from build123d import *

# Parameters (mm, degrees)
SCHIZZO1_W                   = 15
SCHIZZO1_H                   = 76.1
ESTRUSIONE_ESTRUSIONE1_DEPTH = 11
SCHIZZO2_W                   = 15
SCHIZZO2_H                   = 8.2
ESTRUSIONE_ESTRUSIONE2_DEPTH = 62.5
SCHIZZO3_R                   = 7.5
ESTRUSIONE_ESTRUSIONE3_DEPTH = 8.2
SCHIZZO4_R                   = 4
ESTRUSIONE_ESTRUSIONE4_DEPTH = 7
SMUSSO1_SIZE                 = 0.5
SCHIZZO5_W                   = 15
SCHIZZO5_H                   = 8.2
ESTRUSIONE_ESTRUSIONE5_DEPTH = 70
F_3_0_3_DIAMETER_HOLE1_D     = 3
F_3_0_3_DIAMETER_HOLE1_DEPTH = 10
F_3_0_3_DIAMETER_HOLE1_TIP   = 0.901290929
RACCORDO1_R                  = 7.5
RACCORDO2_R                  = 7
F_4_0_4_DIAMETER_HOLE1_D     = 4
SCHIZZO12_R                  = 4.5
ESTRUSIONE_ESTRUSIONE6_DEPTH = 1
F_3_0_3_DIAMETER_HOLE2_D     = 3
F_3_0_3_DIAMETER_HOLE2_DEPTH = 8.2


with BuildPart() as part:
    # Schizzo1 → Estrusione-Estrusione1 (new body)
    with BuildSketch(Plane.XY):
        with Locations((7.5, 38.05)):
            Rectangle(SCHIZZO1_W, SCHIZZO1_H)
    extrude(amount=ESTRUSIONE_ESTRUSIONE1_DEPTH)

    # Schizzo2 → Estrusione-Estrusione2 (add)
    with BuildSketch(Plane.XY.offset(11)):
        with Locations((7.5, 4.1)):
            Rectangle(SCHIZZO2_W, SCHIZZO2_H)
    extrude(amount=ESTRUSIONE_ESTRUSIONE2_DEPTH)

    # Schizzo3 → Estrusione-Estrusione3 (add)
    with BuildSketch(Plane(origin=(0, 8.2, 0), x_dir=(1, 0, 0), z_dir=(0, 1, 0))):
        with Locations((7.5, -73.5)):
            Circle(SCHIZZO3_R)
    extrude(amount=-ESTRUSIONE_ESTRUSIONE3_DEPTH)

    # Schizzo4 → Estrusione-Estrusione4 (add)
    with BuildSketch(Plane(origin=(0, 8.2, 0), x_dir=(1, 0, 0), z_dir=(0, 1, 0))):
        with Locations(Location((7.5, -73.5, 0), (0, 0, 90))):
            Circle(SCHIZZO4_R)
    extrude(amount=ESTRUSIONE_ESTRUSIONE4_DEPTH)

    # Smusso1
    smusso1_edges = [part.edges().sort_by_distance(p)[0] for p in [
        (7.5, 15.2, 77.5),
    ]]
    chamfer(smusso1_edges, length=SMUSSO1_SIZE)

    # Schizzo5 → Estrusione-Estrusione5 (add)
    with BuildSketch(Plane.XY.offset(11)):
        with Locations((7.5, 72)):
            Rectangle(SCHIZZO5_W, SCHIZZO5_H)
    extrude(amount=ESTRUSIONE_ESTRUSIONE5_DEPTH)

    # Ø3.0 (3) Diameter Hole1
    with Locations(Plane(origin=(0, 76.1, 0), x_dir=(1, 0, 0), z_dir=(0, 1, 0))):
        with Locations((7.5, -49.5), (7.5, -53.5)):
            Hole(F_3_0_3_DIAMETER_HOLE1_D / 2, depth=F_3_0_3_DIAMETER_HOLE1_DEPTH)
            with Locations((0, 0, -(F_3_0_3_DIAMETER_HOLE1_DEPTH + F_3_0_3_DIAMETER_HOLE1_TIP / 2))):  # 118° drill point
                Cone(0, F_3_0_3_DIAMETER_HOLE1_D / 2, F_3_0_3_DIAMETER_HOLE1_TIP, mode=Mode.SUBTRACT)

    # Raccordo1
    raccordo1_edges = [part.edges().sort_by_distance(p)[0] for p in [
        (15, 72, 81),
        (0, 72, 81),
    ]]
    fillet(raccordo1_edges, radius=RACCORDO1_R - 0.0001)  # a hair under: the kernel refuses the full size

    # Raccordo2
    raccordo2_edges = [part.edges().sort_by_distance(p)[0] for p in [
        (7.5, 76.1, 0),
        (7.5, 0, 0),
    ]]
    fillet(raccordo2_edges, radius=RACCORDO2_R)

    # Ø4.0 (4) Diameter Hole1 (through all)
    with Locations(Plane(origin=(15, 0, 0), x_dir=(0, 0, -1), z_dir=(1, 0, 0))):
        with Locations((-5.5, 19.8), (-5.5, 47.8)):
            Hole(F_4_0_4_DIAMETER_HOLE1_D / 2)

    # Schizzo12 → Estrusione-Estrusione6 (add)
    with BuildSketch(Plane(origin=(0, 8.2, 0), x_dir=(1, 0, 0), z_dir=(0, 1, 0))):
        with Locations(Location((7.5, -73.5, 0), (0, 0, 90))):
            Circle(SCHIZZO12_R)
    extrude(amount=ESTRUSIONE_ESTRUSIONE6_DEPTH)

    # Ø3.0 (3) Diameter Hole2
    with Locations(Plane(origin=(0, 76.1, 0), x_dir=(1, 0, 0), z_dir=(0, 1, 0))):
        with Locations((7.5, -73.5)):
            Hole(F_3_0_3_DIAMETER_HOLE2_D / 2, depth=F_3_0_3_DIAMETER_HOLE2_DEPTH)


solid = part.part
For this review, take the finished solid that the model builds, in its own axes (mm). A direction names the side the tool comes from. Coordinates: 2 decimals unless noted, no trailing zeros. Loops run counter-clockwise (first coordinate to the right, second up) from the corner with the lowest first, then second, coordinate; pieces in that order, holes last. Notation, with made-up numbers: (72.25, -36) - (105.25, -36) arc R16 cw to (105.25, -8) - close; hole circle Ø2 at (-33.5, 2). An arc over 180 degrees is marked (long way). Use a Markdown table: item, result. Add a question column.
Item 1: Insertion check: pin 1 Ø8 at (x, y) = (3, 51) entering from +Z. The pin has a flat end and moves straight along its axis. Give the tip position at first contact, or say it passes through.
Item 2: We need section B-B (z = 26.5). Give the boundary of the cut face in (x, y), and give its area (3 significant figures).
Item 3: We need section D-D (x = 1.75). Give the boundary of the cut face in (y, z), and give its area (3 significant figures).
Item 4: Tool access review of faces 4 (the face through (7.825, 71.943, 50.964)), 5 (the face through (7, 0, 43)), 6 (the face through (7, 15.2, 74)), 7 (the face through (10, 9.2, 77)), 8 (the face through (7.395, 49.783, 5.24)): name each direction out of +Z, -Z, +X, -X, +Y, -Y from which nothing blocks a thin tool from reaching the whole face with its end or side.
Item 5: For line 1 (Y direction, x = 9, z = 20.5); line 2 (X direction, y = 70, z = 49.5); line 3 (Z direction, x = 7.5, y = 70.25), list the stretches that pass through material, from the lowest coordinate up.
Item 6: We need section C-C (z = 49.5). Give the boundary of the cut face in (x, y).
Item 7: Mouldability with a two-part tool opening along Z and no side actions: class faces 1 (the face through (7, 67.9, 46)), 2 (the face through (6.694, 71.943, 72.235)), 3 (the face through (7.34, 4.16, 81)) as pulls with the +Z half, pulls with the -Z half, needs draft (parallel to the pull), parting line crosses it, or undercut.
Item 8: We need section A-A (y = 47.8). Give the boundary of the cut face in (x, z).
Results list:
| question | item | result |
|---|---|---|
| 1 | pin 1 | stops at z = 11 |
| 2 | outline | (0, 0) - (15, 0) - (15, 8.2) - (0, 8.2) - close; (0, 67.9) - (15, 67.9) - (15, 76.1) - (0, 76.1) - close |
| 2 | area | 246 mm^2 |
| 3 | outline | (0, 7) arc R7 ccw to (7, 0) - (69.1, 0) arc R7 ccw to (76.1, 7) - (76.1, 78.32) - (67.9, 78.32) - (67.9, 11) - (8.2, 11) - (8.2, 78.32) - (0, 78.32) - close; hole circle Ø4 at (19.8, 5.5); hole circle Ø4 at (47.8, 5.5) |
| 3 | area | 1,890 mm^2 |
| 4 | face 4 | +Y |
| 4 | face 5 | +Z, -Z, +X, -X, -Y |
| 4 | face 6 | +Z, +X, -X |
| 4 | face 7 | none |
| 4 | face 8 | +X, -X |
| 5 | line 1 | y = 0 to 8.2, 67.9 to 76.1 |
| 5 | line 2 | x = 0 to 6, 9 to 15 |
| 5 | line 3 | z = 0.1 to 48, 51 to 52, 55 to 72, 75 to 81 |
| 6 | outline | (0, 0) - (15, 0) - (15, 8.2) - (0, 8.2) - close; (0, 67.9) - (6, 67.9) - (6, 76.1) - (0, 76.1) - close; (9, 67.9) - (15, 67.9) - (15, 76.1) - (9, 76.1) - close |
| 7 | face 1 | needs draft |
| 7 | face 2 | undercut |
| 7 | face 3 | pulls with the +Z half |
| 8 | outline | (0, 0) - (15, 0) - (15, 3.5) - (0, 3.5) - close; (0, 7.5) - (15, 7.5) - (15, 11) - (0, 11) - close |
